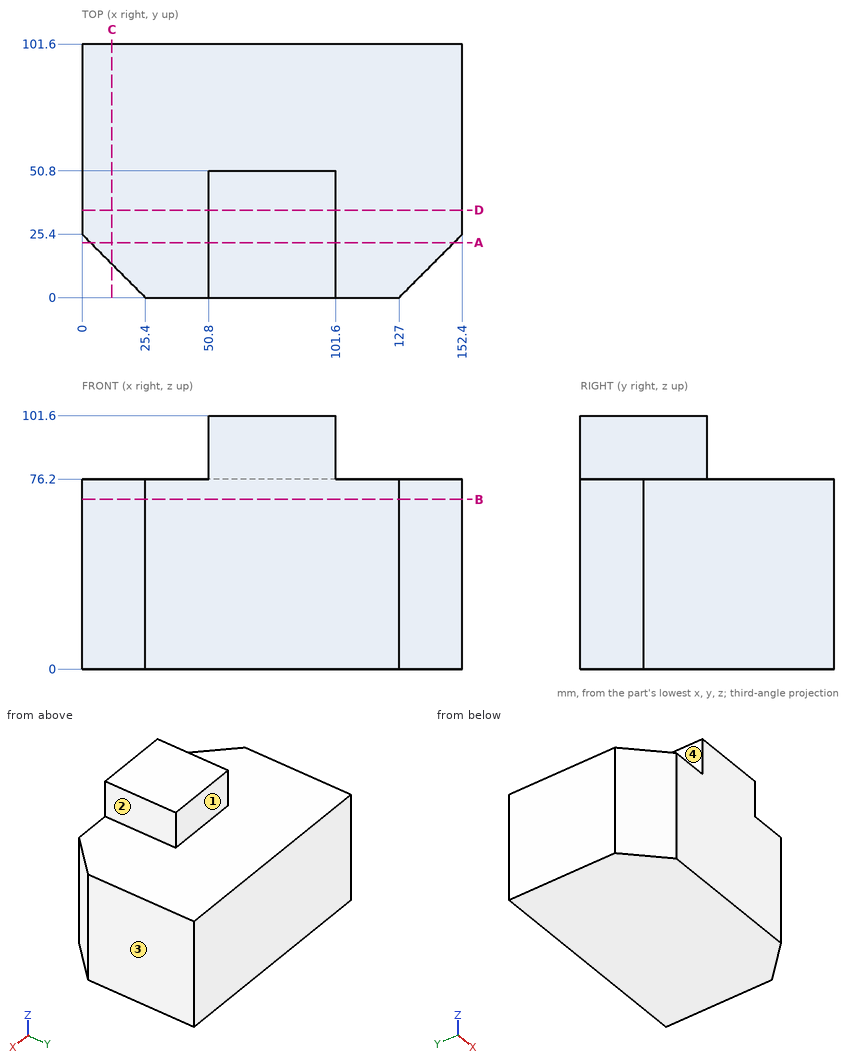
Study the drawing (mm; zero at the part's minimum x, y, z) and answer. A direction names the side the tool comes from. Coordinates: 2 decimals unless noted, no trailing zeros. Loops run counter-clockwise (first coordinate to the right, second up) from the corner with the lowest first, then second, coordinate; pieces in that order, holes last. Notation, with made-up numbers: M -13.5,-5 L -3.5,-5 A10 ccw -3.5,14 Z; hole C 29.5,12.25 d6. An arc over 180 degrees is marked long. Answer as a JSON object with one key per item and string values. Group by question number.
Item 1: Section B-B (z = 68) is taken. Write down the section's boundary in (x, y).
Item 2: Each of these flat-tipped pins is pushed along its axis until it touches: P1, Ø3, axis at y = 17.5, z = 89, coming from the +X side; P2, Ø7.5, axis at y = 28, z = 86, coming from the -X side; P3, Ø7.5, axis at x = 77, z = 90, coming from the +Y side. Where does it stop, or does it pass through?
Item 3: Section C-C (x = 12) is taken. Write down the section's boundary in (y, z).
Item 4: Section A-A (y = 22) is taken. Write down the section's boundary in (x, z).
Item 5: Which of the six approach directions +Z, -Z, +X, -X, +Y, -Y give full straight-line access (tool end or side, diameter ignored) to the marked faces 1, 2, 3 and 4?
Item 6: Section D-D (y = 35) is taken. Write down the section's boundary in (x, z).
Item 7: Consider L1, parallel to Z at x = 118.5, y = 72.5; L2, parallel to Y at x = 24.5, z = 48; L3, parallel to Y at x = 138, z = 69. Determine where each line is inside the solid, lowest interval first.
Solved:
{
 "1": {"outline": "M 0,25.4 L 25.4,0 L 127,0 L 152.4,25.4 L 152.4,101.6 L 0,101.6 Z"},
 "2": {"P1": "stops at x = 101.6", "P2": "stops at x = 50.8", "P3": "stops at y = 50.8"},
 "3": {"outline": "M 13.4,0 L 101.6,0 L 101.6,76.2 L 13.4,76.2 Z"},
 "4": {"outline": "M 3.4,0 L 149,0 L 149,76.2 L 101.6,76.2 L 101.6,101.6 L 50.8,101.6 L 50.8,76.2 L 3.4,76.2 Z"},
 "5": {"face 1": "+Z, +X, -X, +Y", "face 2": "+Z, +X, +Y, -Y", "face 3": "+Z, -Z, +X, +Y, -Y", "face 4": "+Z, -X, +Y, -Y"},
 "6": {"outline": "M 0,0 L 152.4,0 L 152.4,76.2 L 101.6,76.2 L 101.6,101.6 L 50.8,101.6 L 50.8,76.2 L 0,76.2 Z"},
 "7": {"L1": "z = 0 to 76.2", "L2": "y = 0.9 to 101.6", "L3": "y = 11 to 101.6"}
}
